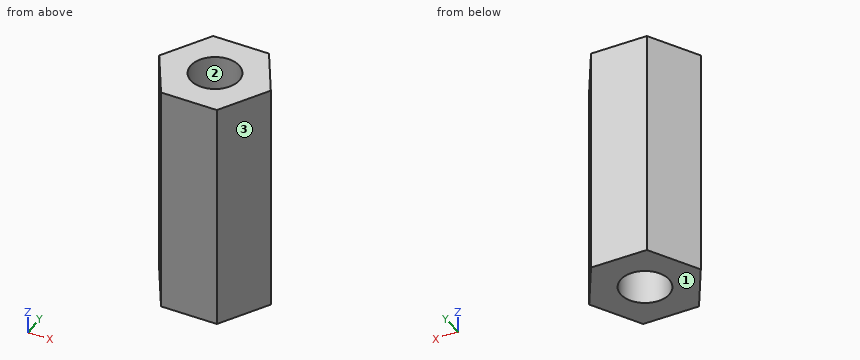
Autodesk Inventor part; units mm, degrees
ref_plane "YZ Plane" through (0, 0, 0) normal (1, 0, 0) x (0, 1, 0)
ref_plane "XZ Plane" through (0, 0, 0) normal (0, 1, 0) x (-1, 0, 0)
ref_plane "XY Plane" through (0, 0, 0) normal (0, 0, 1) x (1, 0, 0)
sketch "Skizze1" plane through (0, 0, 0) normal (0, 0, 1) x (1, 0, 0)
  line L0 (-1.4434, 2.5) -> (1.4434, 2.5)
  line L1 (1.4434, 2.5) -> (2.8868, 0)
  line L2 (2.8868, 0) -> (1.4434, -2.5)
  line L3 (1.4434, -2.5) -> (-1.4434, -2.5)
  line L4 (-1.4434, -2.5) -> (-2.8868, 0)
  line L5 (-2.8868, 0) -> (-1.4434, 2.5)
  point P0 (0, 0)
  point P1 (0, 0)
  point P2 (0, 2.5)
  point P3 (0, -2.5)
  dimension "d3" = 120
  dimension "d4" = 120
  dimension "d5" = 120
  dimension "d6" = 5
extrude "Extrusion1" add sketch "Skizze1" along normal blind 12
sketch "Skizze2" plane through (0, 0, 12) normal (0, 0, 1) x (1, 0, 0)
  point P0 (0, 0)
  point P1 (0, 0)
hole "Bohrung1" at (0, 0, 12) direction (0, 0, -1) diameter 2.5 end through all
thread "Gewinde1"
properties part number "12mm_Innengewinde"
Verification items for the finished model (mm, model axes). Face numbers are marked on the shaded views. Give positions to 0.01 mm unless a question says otherwise; leave off trailing zeros. Write each loop counter-clockwise with the first axis right and the second up, starting at its lowest first coordinate (ties: lowest second). Pieces come first, ordered by that corner, then holes. Notation, with made-up numbers: M 22,82 L 48,82 A26 ccw 48,104 Z; hole C 21.5,53.5 d7. An arc over 180 degrees is marked long. One line per question, with ' | ' between items.
1) Mould release check, pull along Y, two halves, no side actions. Record for the marked faces 1, 2 and 3: released by +Y, released by -Y, zero draft, split by the parting line, or undercut.
Result:
face 1: zero draft | face 2: undercut | face 3: released by -Y
2) Section check C-C on y = -0.7. Enter the section's corners in (x, z).
Result:
outline: M -2.48,0 L -1.04,0 L -1.04,12 L -2.48,12 Z; M 1.04,0 L 2.48,0 L 2.48,12 L 1.04,12 Z
3) Section check B-B on x = -1.1. Enter the section's corners in (y, z), plus the area to 3 significant figures.
Result:
outline: M -2.5,0 L -0.59,0 L -0.59,12 L -2.5,12 Z; M 0.59,0 L 2.5,0 L 2.5,12 L 0.59,12 Z | area: 45.8 mm2
4) Gauge pin test, flat ends, axial feed: pin 1 Ø2 at (x, y) = (0, 0) entering from +Z; pin 2 Ø2 at (y, z) = (0.5, 10.5) entering from -X. Record the tip position at first contact, or that the pin passes through.
Result:
pin 1: passes through | pin 2: stops at x = -2.89
5) Section check D-D on x = 2.2. Enter the section's corners in (y, z).
Result:
outline: M -1.19,0 L 1.19,0 L 1.19,12 L -1.19,12 Z
6) Thickness scan on line 1 along Y through (x, z) = (0, 4.75); line 2 along Y through (x, z) = (-0.8, 7); line 3 along X through (y, z) = (-0.15, 3.5). Record the ranges inside material, lowest first. Write a range as [from, to].
Result:
line 1: y = [-2.5, -1.25], [1.25, 2.5] | line 2: y = [-2.5, -0.96], [0.96, 2.5] | line 3: x = [-2.8, -1.24], [1.24, 2.8]
7) Section check A-A on z = 3.25. Enter the section's corners in (x, y).
Result:
outline: M -2.89,0 L -1.44,-2.5 L 1.44,-2.5 L 2.89,0 L 1.44,2.5 L -1.44,2.5 Z; hole C 0,0 d2.5
